```python
from build123d import *

# Parameters (mm, degrees)
ESQUISSE1_W             = 45
ESQUISSE1_H             = 50
EXTRUSION1_DEPTH        = 11
ESQUISSE2_W             = 10
ESQUISSE2_H             = 48
ENL_V_MAT_EXTRU_1_DEPTH = 10


with BuildPart() as part:
    # Esquisse1 → Extrusion1 (new body)
    with BuildSketch(Plane.XY):
        with Locations((-22.5, 25)):
            Rectangle(ESQUISSE1_W, ESQUISSE1_H)
    extrude(amount=EXTRUSION1_DEPTH)

    # Esquisse2 → Enlèv. mat.-Extru.1 (cut)
    with BuildSketch(Plane.XY.offset(11)):
        with Locations((-39, 25)):
            Rectangle(ESQUISSE2_W, ESQUISSE2_H)
        with Locations((-28, 25)):
            Rectangle(ESQUISSE2_W, ESQUISSE2_H)
        with Locations((-17, 25)):
            Rectangle(ESQUISSE2_W, ESQUISSE2_H)
        with Locations((-6, 25)):
            Rectangle(ESQUISSE2_W, ESQUISSE2_H)
    extrude(amount=-ENL_V_MAT_EXTRU_1_DEPTH, mode=Mode.SUBTRACT)


solid = part.part
```
Geometry check sheet. Reference: the model listing, model coordinates, mm. A direction names the side the tool comes from. Coordinates: 2 decimals unless noted, no trailing zeros. Loops run counter-clockwise (first coordinate to the right, second up) from the corner with the lowest first, then second, coordinate; pieces in that order, holes last. Notation, with made-up numbers: (-37, 39.5) - (12, 39.5) arc R28 cw to (12, 68.5) - close; hole circle Ø3 at (-24.5, 25.5). An arc over 180 degrees is marked (long way). One line per item, written item: value. Start each with the question number.
(1) Cross-section at A-A on z = 6.5. Enter the section's corners in (x, y), plus the area to 3 significant figures.
(2) Depth check by flat-ended pin: P1, Ø3, axis at x = -8.5, y = 16, coming from the +Z side. Enter the tip coordinate at first touch or a pass-through.
(3) Cross-section at B-B on x = -19. Enter the section's corners in (y, z), plus the area to 3 significant figures.
(4) Mould release check, pull along Y, two halves, no side actions. Record for faces 1 (the flat face through (-22.6, 28.8, 11)), 2 (the flat face through (-23, 50, 5)), 3 (the flat face through (-39, 49, 6)): released by +Y, released by -Y, zero draft, split by the parting line, or undercut.
(5) Tool access check on faces 4 (the flat face through (-22, 25, 6)), 5 (the flat face through (-45, 25, 5)). Record the directions out of +Z, -Z, +X, -X, +Y, -Y that give a thin tool (end or side, any length) a straight path to the whole face; none if there is none.
(6) Material ranges on line 1 (X direction, y = 23, z = 10); line 2 (Y direction, x = -8, z = 6.75); line 3 (Z direction, x = -13.5, y = 27.5), recorded low to high. Write a range as [from, to].
(7) Cross-section at C-C on y = 12.5. Enter the section's corners in (x, z).
Results below:
1. outline: (-45, 0) - (0, 0) - (0, 50) - (-45, 50) - close; hole (-44, 1) - (-34, 1) - (-34, 49) - (-44, 49) - close; hole (-33, 1) - (-23, 1) - (-23, 49) - (-33, 49) - close; hole (-22, 1) - (-12, 1) - (-12, 49) - (-22, 49) - close; hole (-11, 1) - (-1, 1) - (-1, 49) - (-11, 49) - close
1. area: 330 mm2
2. P1: stops at z = 1
3. outline: (0, 0) - (50, 0) - (50, 11) - (49, 11) - (49, 1) - (1, 1) - (1, 11) - (0, 11) - close
3. area: 70.0 mm2
4. face 1: zero draft
4. face 2: released by +Y
4. face 3: undercut
5. face 4: +Z
5. face 5: +Z, -Z, -X, +Y, -Y
6. line 1: x = [-45, -44], [-34, -33], [-23, -22], [-12, -11], [-1, 0]
6. line 2: y = [0, 1], [49, 50]
6. line 3: z = [0, 1]
7. outline: (-45, 0) - (0, 0) - (0, 11) - (-1, 11) - (-1, 1) - (-11, 1) - (-11, 11) - (-12, 11) - (-12, 1) - (-22, 1) - (-22, 11) - (-23, 11) - (-23, 1) - (-33, 1) - (-33, 11) - (-34, 11) - (-34, 1) - (-44, 1) - (-44, 11) - (-45, 11) - close
